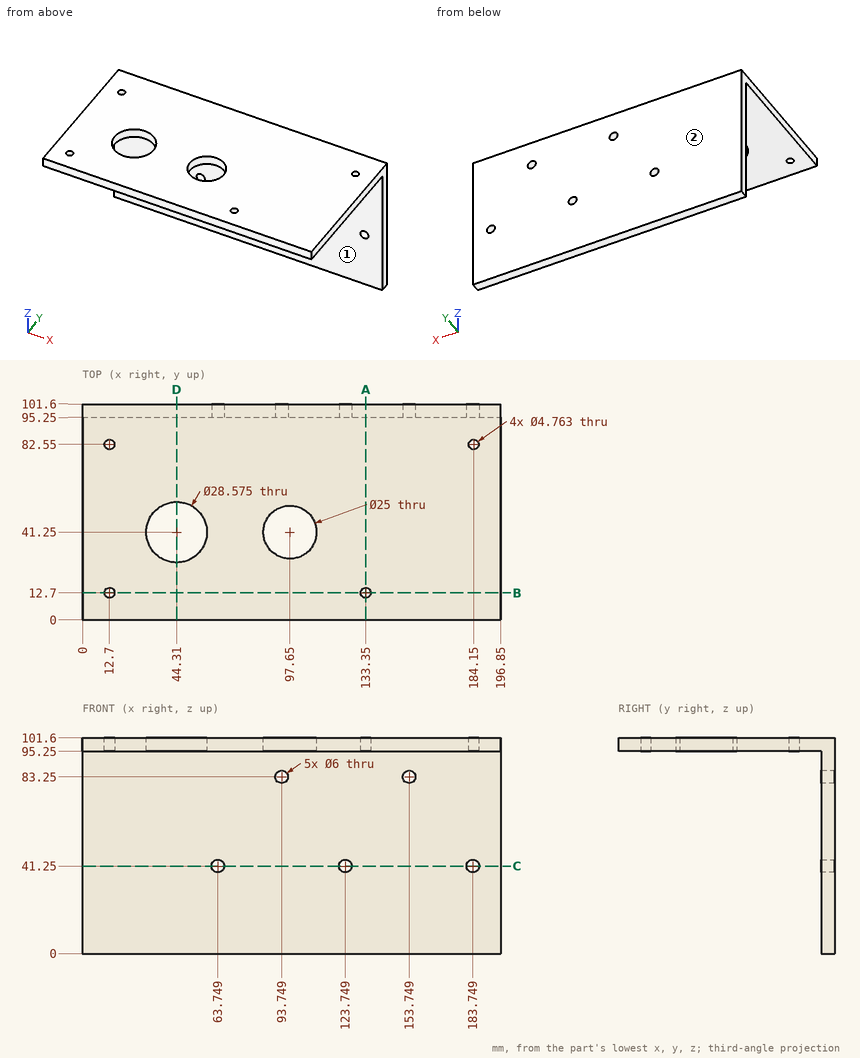
Could you check a few things on this drawing? It's one solid part, dimensions in mm from its lowest x, y, z. A direction names the side the tool comes from. Round coordinates to 2 decimals unless told otherwise and drop trailing zeros. Write each loop counter-clockwise with the first axis right and the second up, starting at its lowest first coordinate (ties: lowest second). Pieces come first, ordered by that corner, then holes. Notation, with made-up numbers: M 72.25,68 L 111.25,68 A20 cw 111.25,99 Z; hole C 4.5,80.25 d4. An arc over 180 degrees is marked long. Answer as CSV lines item,"result". Start each with the question number.
1. Suppose I cut it at C-C on z = 41.25. Write out the boundary of the cut face in (x, y), then the cut area to 3 significant figures.
2. Suppose I cut it at B-B on y = 12.7. Write out the boundary of the cut face in (x, z), then the cut area to 3 significant figures.
3. On a 3-axis mill with a long thin cutter (end or side, diameter ignored), from which of +Z, -Z, +X, -X, +Y, -Y can I reach the whole of each face in a straight line? I mean the marked faces 1 and 2. Say none if no direction works.
4. Suppose I cut it at A-A on x = 133.35. Write out the boundary of the cut face in (y, z), then the cut area to 3 significant figures.
5. I'm going to push flat-ended pins straight in: pin 1 Ø5.5 at (x, z) = (123.75, 41.25) entering from -Y; pin 2 Ø7.5 at (x, y) = (133.35, 12.7) entering from -Z; pin 3 Ø7 at (x, z) = (183.75, 41.25) entering from -Y. Where does each tip first touch, or does it pass through?
6. Suppose I cut it at D-D on x = 44.31. Write out the boundary of the cut face in (y, z).
7. I need wall thicknesses on probe 1 along X at (y, z) = (97, 83); probe 2 along Y at (x, z) = (12.7, 100); probe 3 along X at (y, z) = (97, 83.25). Which ranges of each line are inside material? Lowest first, please.
Check result:
1,outline,"M 0,95.25 L 60.75,95.25 L 60.75,101.6 L 0,101.6 Z; M 66.75,95.25 L 120.75,95.25 L 120.75,101.6 L 66.75,101.6 Z; M 126.75,95.25 L 180.75,95.25 L 180.75,101.6 L 126.75,101.6 Z; M 186.75,95.25 L 196.85,95.25 L 196.85,101.6 L 186.75,101.6 Z"
1,area,"1,140 mm2"
2,outline,"M 0,95.25 L 10.32,95.25 L 10.32,101.6 L 0,101.6 Z; M 15.08,95.25 L 130.97,95.25 L 130.97,101.6 L 15.08,101.6 Z; M 135.73,95.25 L 196.85,95.25 L 196.85,101.6 L 135.73,101.6 Z"
2,area,"1,190 mm2"
3,face 1,"-Z, +X, -X, -Y"
3,face 2,"+Z, -Z, +X, -X, +Y"
4,outline,"M 0,95.25 L 10.32,95.25 L 10.32,101.6 L 0,101.6 Z; M 15.08,95.25 L 95.25,95.25 L 95.25,0 L 101.6,0 L 101.6,101.6 L 15.08,101.6 Z"
4,area,"1,220 mm2"
5,pin 1,"passes through"
5,pin 2,"stops at z = 95.25"
5,pin 3,"stops at y = 95.25"
6,outline,"M 0,95.25 L 26.96,95.25 L 26.96,101.6 L 0,101.6 Z; M 55.54,95.25 L 95.25,95.25 L 95.25,0 L 101.6,0 L 101.6,101.6 L 55.54,101.6 Z"
7,probe 1,"x = 0 to 90.76, 96.74 to 150.76, 156.74 to 196.85"
7,probe 2,"y = 0 to 10.32, 15.08 to 80.17, 84.93 to 101.6"
7,probe 3,"x = 0 to 90.75, 96.75 to 150.75, 156.75 to 196.85"
